Verification items for the finished model (mm, model axes). A direction names the side the tool comes from. Coordinates: 2 decimals unless noted, no trailing zeros. Loops run counter-clockwise (first coordinate to the right, second up) from the corner with the lowest first, then second, coordinate; pieces in that order, holes last. Notation, with made-up numbers: (50.25, -5) -> (63.25, -5) arc R9 cw to (63.25, 1) -> close; hole circle Ø3 at (9.5, 35.5). An arc over 180 degrees is marked (long way). Answer as a JSON object with one key per item and string values. Group by question number.
Q1. Scan lines: L1, parallel to X at y = 9.5, z = 14; L2, parallel to X at y = 0.5, z = 32; L3, parallel to X at y = 3.25, z = -18. Record each from-to range of solid material in increasing order.
Q2. Cross-section at A-A on z = 0. Record the boundary of the cut face in (x, y), and give its area (3 significant figures).
Q3. Cross-section at B-B on x = -197. Record the boundary of the cut face in (y, z).
Q4. Set-up check for faces 5 (the flat face through (-274, 5, -79)), 6 (the flat face through (26, 5, -100)): record each of +Z, -Z, +X, -X, +Y, -Y from which the full face is reachable in a straight line by a thin tool's end or side.
Q5. Release check for a two-part mould opening along Z. For faces 1 (the cylindrical face through (-125.447, 2.465, -83.314)), 2 (the cylindrical face through (-289.89, 5.07, 81.96)), 3 (the flat face through (-124, 5, 71)), 4 (the flat face through (-4, 10, -1)) record: released by +Z, released by -Z, zero draft, split by the parting line, or undercut.
Q6. Gauge pin test, flat ends, axial feed: pin 1 Ø6 at (x, z) = (290.23, -33.23) entering from -Y; pin 2 Ø9 at (x, z) = (-121, -76) entering from -Y; pin 3 Ø6 at (y, z) = (8.5, 74.5) entering from -X. Record the tip position at first contact, or that the pin passes through.
Q7. Cross-section at C-C on y = 1.5. Give the number of separate pieces and of enclosed holes in the cut face, and give its area (3 significant figures).
```python
from build123d import *

# Parameters (mm, degrees)
SKETCH1_W             = 614
SKETCH1_H             = 200
EXTRUDE1_DEPTH        = 10
SKETCH2_R             = 29
SKETCH2_R_2           = 4
EXTRUDE2_DEPTH        = 10
M8_TAPPED_HOLE2_D     = 6.8
M8_TAPPED_HOLE2_DEPTH = 19.75
M8_TAPPED_HOLE2_TIP   = 2.042926105
SKETCH6_R             = 22.5
EXTRUDE3_DEPTH        = 10
SKETCH7_R             = 9
EXTRUDE4_DEPTH        = 5
LPATTERN1_COUNT       = 2
LPATTERN1_PITCH       = 150
LPATTERN1_COUNT_DIR2  = 2
LPATTERN1_PITCH_DIR2  = 150
M8_TAPPED_HOLE3_D     = 6.8
M8_TAPPED_HOLE3_DEPTH = 19.75
M8_TAPPED_HOLE3_TIP   = 2.042926105
FILLET1_R             = 60


with BuildPart() as part:
    # Sketch1 → Extrude1 (new body)
    with BuildSketch(Plane(origin=(0, 0, 0), x_dir=(1, 0, 0), z_dir=(0, 1, 0))):
        Rectangle(SKETCH1_W, SKETCH1_H)
    extrude(amount=EXTRUDE1_DEPTH)

    # Sketch2 → Extrude2 (cut)
    with BuildSketch(Plane(origin=(0, 10, 0), x_dir=(1, 0, 0), z_dir=(0, 1, 0))):
        with Locations(Location((-197, 0, 0), (0, 0, 270))):
            Circle(SKETCH2_R)
        with Locations(Location((-272, 75, 0), (0, 0, 270))):
            Circle(SKETCH2_R_2)
        with Locations(Location((-122, 75, 0), (0, 0, 90))):
            Circle(SKETCH2_R_2)
        with Locations(Location((-122, -75, 0), (0, 0, 270))):
            Circle(SKETCH2_R_2)
        with Locations(Location((-272, -75, 0), (0, 0, 90))):
            Circle(SKETCH2_R_2)
    extrude(amount=-EXTRUDE2_DEPTH, mode=Mode.SUBTRACT)

    # M8 Tapped Hole2
    with Locations(Plane(origin=(223.765981284, 10, -33.234018716), x_dir=(0, 0, 1), z_dir=(0, 1, 0))):
        with Locations((0, 0), (0, 66.468037432), (66.468037432, 0), (66.468037432, 66.468037432)):
            Hole(M8_TAPPED_HOLE2_D / 2, depth=M8_TAPPED_HOLE2_DEPTH)
            with Locations((0, 0, -(M8_TAPPED_HOLE2_DEPTH + M8_TAPPED_HOLE2_TIP / 2))):  # 118° drill point
                Cone(0, M8_TAPPED_HOLE2_D / 2, M8_TAPPED_HOLE2_TIP, mode=Mode.SUBTRACT)

    # Sketch6 → Extrude3 (cut)
    with BuildSketch(Plane(origin=(0, 10, 0), x_dir=(1, 0, 0), z_dir=(0, 1, 0))):
        with Locations(Location((244, 0, 0), (0, 0, 270))):
            Circle(SKETCH6_R)
    extrude(amount=-EXTRUDE3_DEPTH, mode=Mode.SUBTRACT)

    # Sketch7 → Extrude4 (cut)
    with BuildSketch(Plane.XZ):
        with Locations(Location((-272, 75, 0), (0, 0, 270))):
            Circle(SKETCH7_R)
    extrude4 = extrude(amount=-EXTRUDE4_DEPTH, mode=Mode.SUBTRACT)

    # LPattern1: Extrude4 2 × 2
    with Locations(*[(i * LPATTERN1_PITCH, 0, -j * LPATTERN1_PITCH_DIR2) for i in range(LPATTERN1_COUNT) for j in range(LPATTERN1_COUNT_DIR2) if (i, j) != (0, 0)]):
        add(extrude4, mode=Mode.SUBTRACT)

    # M8 Tapped Hole3
    with Locations(Plane(origin=(42, 10, -18), x_dir=(0, 0, 1), z_dir=(0, 1, 0))):
        with Locations((0, 0), (0, 36), (36, 0), (36, 36)):
            Hole(M8_TAPPED_HOLE3_D / 2, depth=M8_TAPPED_HOLE3_DEPTH)
            with Locations((0, 0, -(M8_TAPPED_HOLE3_DEPTH + M8_TAPPED_HOLE3_TIP / 2))):  # 118° drill point
                Cone(0, M8_TAPPED_HOLE3_D / 2, M8_TAPPED_HOLE3_TIP, mode=Mode.SUBTRACT)

    # Fillet1
    fillet1_edges = [part.edges().sort_by_distance(p)[0] for p in [
        (-307, 5, -100),
        (-307, 5, 100),
    ]]
    fillet(fillet1_edges, radius=FILLET1_R)


solid = part.part
```
Computed values:
{
 "1": {"L1": "x = -307 to -222.4, -171.6 to 226.39, 261.61 to 307", "L2": "x = -307 to 220.6, 226.93 to 287.07, 293.4 to 307", "L3": "x = -307 to -219.74, -174.26 to 38.6, 45.4 to 74.6, 81.4 to 230.5, 257.5 to 307"},
 "2": {"outline": "(-307, 0) -> (-226, 0) -> (-226, 10) -> (-307, 10) -> close; (-168, 0) -> (221.5, 0) -> (221.5, 10) -> (-168, 10) -> close; (266.5, 0) -> (307, 0) -> (307, 10) -> (266.5, 10) -> close", "area": "5,110 mm²"},
 "3": {"outline": "(0, -100) -> (10, -100) -> (10, -29) -> (0, -29) -> close; (0, 29) -> (10, 29) -> (10, 100) -> (0, 100) -> close"},
 "4": {"face 5": "-Y", "face 6": "-Z, +X, -X, +Y, -Y"},
 "5": {"face 1": "undercut", "face 2": "released by +Z", "face 3": "undercut", "face 4": "zero draft"},
 "6": {"pin 1": "passes through", "pin 2": "stops at y = 5", "pin 3": "stops at x = -298.07"},
 "7": {"separate pieces": "1", "enclosed holes": "14", "area": "116,000 mm²"}
}
